Verification items for the finished model (mm, model axes). A direction names the side the tool comes from. Coordinates: 2 decimals unless noted, no trailing zeros. Order: outer loops, then holes, each group sorted by start corner. A loop starts at its lowest first (then second) coordinate and runs counter-clockwise, first axis right, second up.
Q1. Set-up check for faces 1 (the flat face through (-273, -50.8, 225)), 2 (the cylindrical face through (-255.84, -24.16, 225.4)): record each of +Z, -Z, +X, -X, +Y, -Y from which the full face is reachable in a straight line by a thin tool's end or side.
Q2. Cross-section at C-C, the plane x = -55. Record the boundary of the cut face in (y, z).
Q3. Cross-section at D-D, the plane y = -6. Record the boundary of the cut face in (x, z).
Q4. Thickness scan on line 1 (Y direction, x = -10, z = 419); line 2 (X direction, y = -28.5, z = 137.5); line 3 (X direction, y = -29.5, z = 59.5). Record the ranges inside material, lowest first.
Q5. Draft check along X on faces 3 (the cylindrical face through (-264.124, -14.486, 225.4)), 4 (the cylindrical face through (255.84, -24.16, 225.4)), 5 (the flat face through (-1, -12, 457.2)), 6 (the cylindrical face through (264.124, -14.486, 225.4)). Enter one of: pulls with the +X half, pulls with the -X half, needs draft (parallel to the pull), parting line crosses it, or undercut.
Q6. Cross-section at B-B, the plane z = 308. Record the boundary of the cut face in (x, y).
Q7. Cross-section at A-A, the plane y = -34.5. Record the boundary of the cut face in (x, z), and give its area (3 significant figures).
Q8. Depth check by flat-ended pin: P1, Ø4, axis at x = -114.5, z = 214.5, coming from the -Y side; P2, Ø12, axis at x = 104.5, y = -23.5, coming from the +Z side; P3, Ø3, axis at y = -45.5, z = 315.5, coming from the -X side; P4, Ø4, axis at y = -11, z = 386.5, coming from the -X side. Enter the tip coordinate at first touch or a pass-through.
from build123d import *

# Parameters (mm, degrees)
EXTRUDE_THIN1_DEPTH = 457.2


with BuildPart() as part:
    # Sketch1 → Extrude-Thin1 (new body)
    with BuildSketch(Plane.XY):
        with BuildLine():
            Line((0, 0), (228.6, 0))
            ThreePointArc((228.6, 0), (264.521024484, -14.878975516), (279.4, -50.8))
            Line((279.4, -50.8), (266.7, -50.8))
            ThreePointArc((266.7, -50.8), (255.540768363, -23.859231637), (228.6, -12.7))
            Line((228.6, -12.7), (0, -12.7))
            Line((0, -12.7), (0, 0))
        make_face()
    extrude_thin1 = extrude(amount=EXTRUDE_THIN1_DEPTH)

    # Mirror1: Extrude-Thin1 across plane
    add(extrude_thin1.mirror(Plane(origin=(0, -12.7, 457.2), x_dir=(0, 0, 1), z_dir=(-1, 0, 0))))


solid = part.part
Check values:
1. face 1: +Z, -Z, +X, -X, -Y
1. face 2: +Z, -Z, -Y
2. outline: (-12.7, 0) - (0, 0) - (0, 457.2) - (-12.7, 457.2) - close
3. outline: (-252.55, 0) - (252.55, 0) - (252.55, 457.2) - (-252.55, 457.2) - close
4. line 1: y = -12.7 to 0
4. line 2: x = -274.24 to -259.49, 259.49 to 274.24
4. line 3: x = -274.72 to -260.19, 260.19 to 274.72
5. face 3: pulls with the -X half
5. face 4: undercut
5. face 5: needs draft
5. face 6: pulls with the +X half
6. outline: (-279.4, -50.8) - (-266.7, -50.8) arc R38.1 cw to (-228.6, -12.7) - (228.6, -12.7) arc R38.1 cw to (266.7, -50.8) - (279.4, -50.8) arc R50.8 ccw to (228.6, 0) - (-228.6, 0) arc R50.8 ccw to start
7. outline: (-276.71, 0) - (-263.04, 0) - (-263.04, 457.2) - (-276.71, 457.2) - close; (263.04, 0) - (276.71, 0) - (276.71, 457.2) - (263.04, 457.2) - close
7. area: 12,500 mm2
8. P1: stops at y = -12.7
8. P2: passes through
8. P3: stops at x = -279.26
8. P4: stops at x = -262.54
